Geometry check sheet. Reference: the model listing, model coordinates, mm. Face numbers are marked on the shaded views. A direction names the side the tool comes from. Give positions to 0.01 mm unless a question says otherwise; leave off trailing zeros. Write each loop counter-clockwise with the first axis right and the second up, starting at its lowest first coordinate (ties: lowest second). Pieces come first, ordered by that corner, then holes. Notation, with made-up numbers: M 42,63.25 L 99,63.25 A13 cw 99,84.25 Z; hole C 89,89 d4. An arc over 180 degrees is marked long. One line per item, written item: value. Start each with the question number.
1. Cross-section at C-C on z = 5.75. Record the cut outline in (x, y), then the cut area to 3 significant figures.
2. Tool access check on the marked faces 3 and 4. Record the directions out of +Z, -Z, +X, -X, +Y, -Y that give a thin tool (end or side, any length) a straight path to the whole face; none if there is none.
3. Cross-section at D-D on y = 154.5. Record the cut outline in (x, z), then the cut area to 3 significant figures.
4. Cross-section at B-B on y = 116. Record the cut outline in (x, z).
5. Cross-section at A-A on x = 0. Record the cut outline in (y, z), then the cut area to 3 significant figures.
6. Release check for a two-part mould opening along X. For the marked faces 1 and 2 record: pulls with the +X half, pulls with the -X half, needs draft (parallel to the pull), parting line crosses it, or undercut.
7. Scan lines: line 1 (Y direction, x = 0, z = 8.25); line 2 (X direction, y = 185, z = 3.75); line 3 (X direction, y = 102.5, z = 8). Record each from-to range of solid material in increasing order.
8. Gauge pin test, flat ends, axial feed: pin 1 (5 mm diameter, centred on x = -3, y = 114.5, fed in from -Z); pin 2 (2 mm diameter, centred on y = 74, z = 1, fed in from +X); pin 3 (2 mm diameter, centred on y = 148.5, z = 1, fed in from -X). Record the tip position at first contact, or that the pin passes through.
from build123d import *

# Parameters (mm, degrees)
SZKIC1_W                    = 40
SZKIC1_H                    = 180
DODANIE_WYCI_GNI_CIE1_DEPTH = 10
SZKIC2_W                    = 5
SZKIC2_H                    = 2.5
WYTNIJ_WYCI_GNI_CIE1_DEPTH  = 182.383571472
SFAZOWANIE1_SIZE            = 1


with BuildPart() as part:
    # Szkic1 → Dodanie-wyciągnięcie1 (new body)
    with BuildSketch(Plane.XY):
        with Locations((0, 110)):
            Rectangle(SZKIC1_W, SZKIC1_H)
        with BuildLine():
            Line((1.493515455, 193.580554333), (-1.493515455, 193.580554333))
            Line((-1.493515455, 193.580554333), (-1.493515455, 192.349789901))
            ThreePointArc((-1.493515455, 192.349789901), (0, 177.5), (1.493515455, 192.349789901))
            Line((1.493515455, 192.349789901), (1.493515455, 193.580554333))
        make_face(mode=Mode.SUBTRACT)
        with BuildLine():
            Line((5, 140), (5, 30))
            ThreePointArc((5, 30), (0, 25), (-5, 30))
            Line((-5, 30), (-5, 140))
            ThreePointArc((-5, 140), (0, 145), (5, 140))
        make_face(mode=Mode.SUBTRACT)
    extrude(amount=DODANIE_WYCI_GNI_CIE1_DEPTH)

    # Szkic2 → Wytnij-wyciągnięcie1 (cut, through all)
    with BuildSketch(Plane(origin=(0, 200, 0), x_dir=(1, 0, 0), z_dir=(0, 1, 0))):
        with Locations((-17.5, -1.25)):
            Rectangle(SZKIC2_W, SZKIC2_H)
        with Locations((17.5, -1.25)):
            Rectangle(SZKIC2_W, SZKIC2_H)
    extrude(amount=-WYTNIJ_WYCI_GNI_CIE1_DEPTH, mode=Mode.SUBTRACT)

    # Sfazowanie1
    sfazowanie1_edges = [part.edges().sort_by_distance(p)[0] for p in [
        (0, 145, 0),
        (-5, 85, 0),
        (0, 25, 0),
        (5, 85, 0),
        (0, 145, 10),
        (-5, 85, 10),
        (0, 25, 10),
        (5, 85, 10),
    ]]
    chamfer(sfazowanie1_edges, length=SFAZOWANIE1_SIZE)


solid = part.part
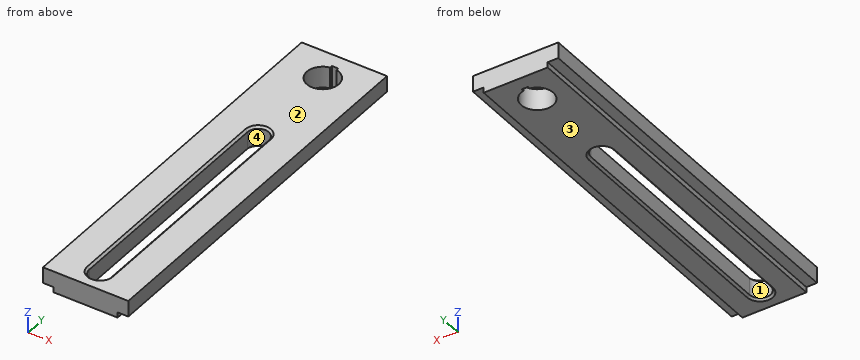
Report:
1. outline: M -20,20 L 20,20 L 20,200 L -20,200 Z; hole M -5,30 A5 ccw 5,30 L 5,140 A5 ccw -5,140 Z; hole M -1.49,192.35 A7.5 ccw long 1.49,192.35 L 1.49,193.58 L -1.49,193.58 Z
1. area: 5,840 mm^2
2. face 3: -Z, +X, -X, +Y, -Y
2. face 4: +Z, -Z
3. outline: M -20,2.5 L -15,2.5 L -15,0 L 15,0 L 15,2.5 L 20,2.5 L 20,10 L -20,10 Z
3. area: 375 mm^2
4. outline: M -20,2.5 L -15,2.5 L -15,0 L -6,0 L -5,1 L -5,9 L -6,10 L -20,10 Z; M 5,1 L 6,0 L 15,0 L 15,2.5 L 20,2.5 L 20,10 L 6,10 L 5,9 Z
5. outline: M 20,0 L 24,0 L 25,1 L 25,9 L 24,10 L 20,10 Z; M 145,1 L 146,0 L 177.5,0 L 177.5,10 L 146,10 L 145,9 Z; M 193.58,0 L 200,0 L 200,10 L 193.58,10 Z
5. area: 437 mm^2
6. face 1: undercut
6. face 2: needs draft
7. line 1: y = 20 to 25, 145 to 177.5, 193.58 to 200
7. line 2: x = -20 to -7.5, 7.5 to 20
7. line 3: x = -20 to -5, 5 to 20
8. pin 1: stops at z = 0.5
8. pin 2: stops at x = 15
8. pin 3: stops at x = -15
